Geometry check sheet. Reference: the model listing, model coordinates, mm. Face numbers are marked on the shaded views. A direction names the side the tool comes from. Round coordinates to 2 decimals unless told otherwise and drop trailing zeros. Order: outer loops, then holes, each group sorted by start corner. A loop starts at its lowest first (then second) coordinate and runs counter-clockwise, first axis right, second up.
```python
from build123d import *

# Parameters (mm, degrees)
EXTRUDE_1_DEPTH     = 18
SKETCH_2_R          = 2.5
CUT_EXTRUDE_1_DEPTH = 73.965745388
SKETCH_3_R          = 2.5
CUT_EXTRUDE_2_DEPTH = 73.965745388


with BuildPart() as part:
    # 草图1 → 凸台-拉伸1 (new body)
    with BuildSketch(Plane.XY):
        Polygon((32, 8), (50, 8), (50, 0), (0, 0), (0, 50), (8, 50), (8, 32), align=None)
    extrude(amount=EXTRUDE_1_DEPTH)

    # 草图2 → 切除-拉伸1 (cut, through all)
    with BuildSketch(Plane.XZ):
        with Locations(Location((40, 9, 0), (0, 0, 270))):
            Circle(SKETCH_2_R)
    extrude(amount=-CUT_EXTRUDE_1_DEPTH, mode=Mode.SUBTRACT)

    # 草图3 → 切除-拉伸2 (cut, through all)
    with BuildSketch(Plane.ZY):
        with Locations(Location((9, 40, 0), (0, 0, 270))):
            Circle(SKETCH_3_R)
    extrude(amount=-CUT_EXTRUDE_2_DEPTH, mode=Mode.SUBTRACT)


solid = part.part
```
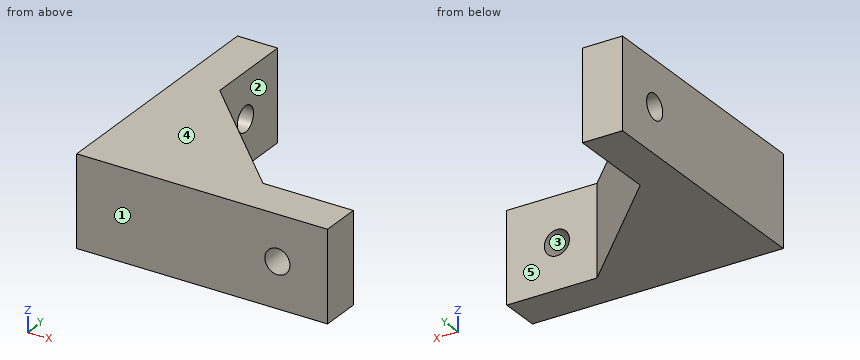
(1) Material ranges on line 1 (X direction, y = 3, z = 9); line 2 (Z direction, x = 3, y = 40); line 3 (X direction, y = 36, z = 14.25), recorded low to high.
Returned:
line 1: x = 0 to 37.5, 42.5 to 50
line 2: z = 0 to 6.5, 11.5 to 18
line 3: x = 0 to 8
(2) Depth check by flat-ended pin: P1, Ø4, axis at x = 41.5, z = 3, coming from the +Y side; P2, Ø6, axis at x = 40, z = 9, coming from the -Y side; P3, Ø10, axis at x = 18.5, z = 12.5, coming from the +Y side; P4, Ø1, axis at x = 16.5, z = 3, coming from the +Y side. Enter the tip coordinate at first touch or a pass-through.
Returned:
P1: stops at y = 8
P2: stops at y = 0
P3: stops at y = 26.5
P4: stops at y = 24
(3) Sectioned sample at A-A, the plane z = 9. Record the cut outline in (x, y), and give its area (3 significant figures).
Returned:
outline: (0, 0) - (37.5, 0) - (37.5, 8) - (32, 8) - (8, 32) - (8, 37.5) - (0, 37.5) - close; (0, 42.5) - (8, 42.5) - (8, 50) - (0, 50) - close; (42.5, 0) - (50, 0) - (50, 8) - (42.5, 8) - close
area: 944 mm2
(4) Set-up check for the marked faces 1 and 2: record each of +Z, -Z, +X, -X, +Y, -Y from which the full face is reachable in a straight line by a thin tool's end or side.
Returned:
face 1: +Z, -Z, +X, -X, -Y
face 2: +Z, -Z, +X, +Y
(5) Sectioned sample at D-D, the plane z = 15. Record the cut outline in (x, y).
Returned:
outline: (0, 0) - (50, 0) - (50, 8) - (32, 8) - (8, 32) - (8, 50) - (0, 50) - close
(6) Sectioned sample at B-B, the plane y = 40. Record the cut outline in (x, z), and give its area (3 significant figures).
Returned:
outline: (0, 0) - (8, 0) - (8, 6.5) - (0, 6.5) - close; (0, 11.5) - (8, 11.5) - (8, 18) - (0, 18) - close
area: 104 mm2
(7) Draft check along Z on the marked faces 3, 4 and 5. Enter one of: released by +Z, released by -Z, zero draft, split by the parting line, or undercut.
Returned:
face 3: undercut
face 4: released by +Z
face 5: zero draft
